Read the model definition and answer for the solid it produces. Units are mm, in the model's axes. Face numbers are marked on the shaded views. Round coordinates to 2 decimals unless told otherwise and drop trailing zeros. Order: outer loops, then holes, each group sorted by start corner. A loop starts at its lowest first (then second) coordinate and runs counter-clockwise, first axis right, second up. Notation, with made-up numbers: (30.5, 85) - (89.5, 85) arc R31 cw to (89.5, 116) - close; hole circle Ø7 at (58, 39). An arc over 180 degrees is marked (long way). Put each result on its own line as item: value. Start each with the question number.
Q1. Section B-B on z = 74 is taken. Give the vertices of the cut face in (x, y).
Q2. Section A-A on z = 29 is taken. Give the vertices of the cut face in (x, y).
Q3. For a pull along X with two mould halves and no side action, classify the marked faces 1 and 2 as pulls with the +X half, pulls with the -X half, needs draft (parallel to the pull), parting line crosses it, or undercut.
Q4. Find the intervals of material crossed by line 1 along Y through (x, z) = (0.25, 15) (3 decimals); line 2 along Y through (x, z) = (5.5, 16), in increasing order. Write a range as from..to.
Q5. Each of these flat-tipped pins is pushed along its axis until it touches: pin 1 Ø8 at (x, y) = (-7.5, 4) entering from -Z; pin 2 Ø1 at (y, z) = (-2, 33.5) entering from -X; pin 3 Ø1.5 at (x, y) = (4, -0.5) entering from -Z; pin 4 Ø8 at (x, z) = (-4.5, 26) entering from +Y. Where does it stop, or does it pass through?
from build123d import *

# Parameters (mm, degrees)
F0_R     = 10
F1_DEPTH = 80
F2_SIZE2 = 4.3744331763
F2_SIZE  = 50
F3_SIZE  = 5
F5_D     = 12.5
F5_DEPTH = 30
F5_TIP   = 3.7553788689


with BuildPart() as f1:
    # F0 (on Top) → F1 (new body)
    with BuildSketch(Plane.XY):
        Circle(F0_R)
    extrude(amount=F1_DEPTH)

    # F2
    f2_edges = [f1.edges().sort_by_distance(p)[0] for p in [
        (-10, 0, 80),
    ]]
    f2_side = f1.faces().sort_by_distance((-10, 0, 40))[0]
    chamfer(f2_edges, length=F2_SIZE, length2=F2_SIZE2, reference=f2_side)

    # F3
    f3_edges = [f1.edges().sort_by_distance(p)[0] for p in [
        (-5.625567, 0, 80),
    ]]
    chamfer(f3_edges, length=F3_SIZE)

    # F5
    with Locations(Plane(origin=(0, 0, 0), x_dir=(1, 0, 0), z_dir=(0, 0, -1))):
        with Locations((0, 0)):
            Hole(F5_D / 2, depth=F5_DEPTH)
            with Locations((0, 0, -(F5_DEPTH + F5_TIP / 2))):  # 118° drill point
                Cone(0, F5_D / 2, F5_TIP, mode=Mode.SUBTRACT)


solid = f1.part
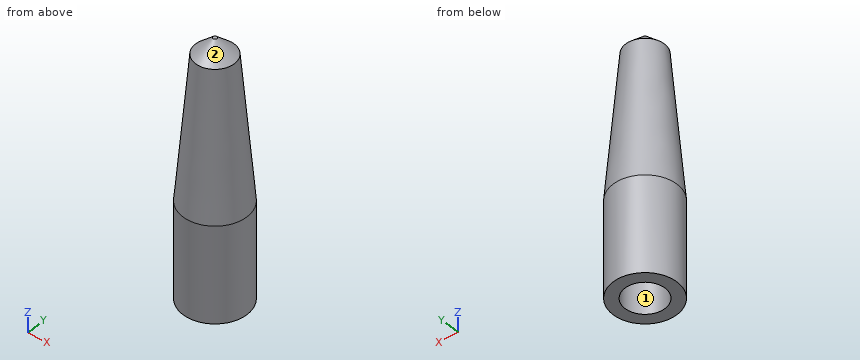
Findings:
1. outline: circle Ø12.3 at (0, 0)
2. outline: circle Ø20 at (0, 0); hole circle Ø12.5 at (0, 0)
3. face 1: undercut
3. face 2: parting line crosses it
4. line 1: -9.997..-6.245, 6.245..9.997
4. line 2: -8.35..-2.97, 2.97..8.35
5. pin 1: z = 0
5. pin 2: x = -9.59
5. pin 3: z = 30.88
5. pin 4: y = 9.99
